from build123d import *

# Parameters (mm, degrees)
F0_W     = 1500
F0_H     = 800
F0_W_2   = 675
F0_H_2   = 325
F1_DEPTH = 125
F2_W     = 675
F2_H     = 325
F3_DEPTH = 1.5


with BuildPart() as f1:
    # F0 (on Top) → F1 (new body, symmetric)
    with BuildSketch(Plane.XY):
        Rectangle(F0_W, F0_H)
        with Locations((-362.5, -187.5)):
            Rectangle(F0_W_2, F0_H_2, mode=Mode.SUBTRACT)
        with Locations((362.5, -187.5)):
            Rectangle(F0_W_2, F0_H_2, mode=Mode.SUBTRACT)
        with Locations((-362.5, 187.5)):
            Rectangle(F0_W_2, F0_H_2, mode=Mode.SUBTRACT)
        with Locations((362.5, 187.5)):
            Rectangle(F0_W_2, F0_H_2, mode=Mode.SUBTRACT)
    extrude(amount=F1_DEPTH, both=True)

    # F2 (on Top) → F3 (join, symmetric)
    with BuildSketch(Plane.XY):
        with Locations((-363.586962, 191.032607)):
            Rectangle(F2_W, F2_H)
        with Locations((361.956573, 184.51087)):
            Rectangle(F2_W, F2_H)
        with Locations((-365.217397, -190.489137)):
            Rectangle(F2_W, F2_H)
        with Locations((361.956573, -187.228256)):
            Rectangle(F2_W, F2_H)
    extrude(amount=F3_DEPTH, both=True)


solid = f1.part
Source: CAD feature listing. Evaluate the final solid. Frame: model axes, mm. A direction names the side the tool comes from. Coordinates: 2 decimals unless noted, no trailing zeros. Loops run counter-clockwise (first coordinate to the right, second up) from the corner with the lowest first, then second, coordinate; pieces in that order, holes last. Notation, with made-up numbers: (44.5, 84) - (73.5, 84) arc R24 cw to (73.5, 108) - close; hole circle Ø8 at (21.5, -31.5). An arc over 180 degrees is marked (long way). Return JSON: item names as keys, results as strings.
Q1. Access query for faces 1 (the flat face through (-25, 185, 2)), 2 (the flat face through (358, 188, 1.5)), 3 (the flat face through (358, 188, -1.5)). Directions: +Z, -Z, +X, -X, +Y, -Y. A direction counts if a zero-diameter tool reaches every point of the face in a straight line with its end or side. Return the directions, or none.
Results:
{"face 1": "+Z, -Z", "face 2": "+Z", "face 3": "-Z"}
Q2. Material intervals for line 1 along X through (y, z) = (-167, 49.5); line 2 along Y through (x, z) = (633, 38); line 3 along Z through (x, y) = (45.5, 46), sorted ascending.
Results:
{"line 1": "-750 to -700, -25 to 25, 700 to 750", "line 2": "-400 to -350, -25 to 25, 350 to 400", "line 3": "-1.5 to 1.5"}
Q3. Section A-A, the plane y = 126. Return loops of the section in (x, z).
Results:
{"outline": "(-750, -125) - (-700, -125) - (-700, -1.5) - (-26.09, -1.5) - (-26.09, 1.5) - (-700, 1.5) - (-700, 125) - (-750, 125) - close; (-25, -125) - (25, -125) - (25, -1.5) - (699.46, -1.5) - (699.46, 1.5) - (25, 1.5) - (25, 125) - (-25, 125) - close; (700, -125) - (750, -125) - (750, 125) - (700, 125) - close"}
Q4. Section B-B, the plane x = 77.5. Return loops of the section in (y, z), plus the area to 3 significant figures.
Results:
{"outline": "(-400, -125) - (-350, -125) - (-350, 125) - (-400, 125) - close; (-349.73, -1.5) - (-25, -1.5) - (-25, -125) - (25, -125) - (25, -1.5) - (347.01, -1.5) - (347.01, 1.5) - (25, 1.5) - (25, 125) - (-25, 125) - (-25, 1.5) - (-349.73, 1.5) - close; (350, -125) - (400, -125) - (400, 125) - (350, 125) - close", "area": "39,400 mm2"}
Q5. Section C-C, the plane z = -77.5. Return loops of the section in (x, y), plus the area to 4 significant figures.
Results:
{"outline": "(-750, -400) - (750, -400) - (750, 400) - (-750, 400) - close; hole (-700, -350) - (-25, -350) - (-25, -25) - (-700, -25) - close; hole (-700, 25) - (-25, 25) - (-25, 350) - (-700, 350) - close; hole (25, -350) - (700, -350) - (700, -25) - (25, -25) - close; hole (25, 25) - (700, 25) - (700, 350) - (25, 350) - close", "area": "322,500 mm2"}
Q6. Contact query for flat-ended pins moving along their axis: P1, Ø6, axis at x = -82, y = 91.5, coming from the -Z side; P2, Ø5, axis at x = 293, y = 151.5, coming from the +Z side. Output: stop coordinate, or through.
Results:
{"P1": "z = -1.5", "P2": "z = 1.5"}
